Build history of the part. All positions in model axes, mm. A direction names the side the tool comes from. Round coordinates to 2 decimals unless told otherwise and drop trailing zeros. Order: outer loops, then holes, each group sorted by start corner. A loop starts at its lowest first (then second) coordinate and runs counter-clockwise, first axis right, second up. Notation, with made-up numbers: (35, 66) -> (74, 66) arc R18 cw to (74, 78) -> close; hole circle Ø9 at (19.5, 86.25). An arc over 180 degrees is marked (long way). Write item = value, one per line.
from build123d import *

# Parameters (mm, degrees)
SKETCH1_W               = 50
SKETCH1_H               = 18.4
BOSS_EXTRUDE1_DEPTH     = 43
SKETCH2_W               = 7.5
SKETCH2_H               = 5
SKETCH2_W_2             = 30
SKETCH2_H_2             = 1.8
CUT_EXTRUDE1_DEPTH      = 15.6
CUT_EXTRUDE2_START      = -22.5
CUT_EXTRUDE2_DEPTH      = 22.5
CUT_EXTRUDE3_START      = -15
CUT_EXTRUDE3_DEPTH      = 15
BOSS_EXTRUDE3_DEPTH     = 7.5
BOSS_EXTRUDE4_START     = 45
BOSS_EXTRUDE4_DEPTH     = 7.5
BOSS_EXTRUDE7_DEPTH     = 30
MTRL_RMV_DEPTH          = 60.694974663
SKETCH22_W              = 36
SKETCH22_H              = 24.066709319
SKETCH22_W_2            = 3
SKETCH22_H_2            = 2.783290681
BOSS_EXTRUDE8_DEPTH     = 2
BOSS_EXTRUDE9_DEPTH     = 36
SKETCH27_W              = 3
SKETCH27_H              = 21.1
BOSS_EXTRUDE10_DEPTH    = 14.25
SKETCH28_R              = 1.5
CUT_EXTRUDE4_DEPTH      = 53.451549072
SKETCH4_W               = 30
SKETCH4_H               = 11
WIRE_HOLE_DEPTH         = 2.5
SKETCH13_W              = 2
SKETCH13_H              = 2
FRONT_SHIELD_PEGS_DEPTH = 3.175
SKETCH14_W              = 2
SKETCH14_H              = 2
TOP_SHIELD_PEGS_DEPTH   = 3.175
FILLET9_R               = 10
FILLET10_R              = 2
LEGS_START              = 24
LEGS_DEPTH              = 12.7
SKETCH29_W              = 2
SKETCH29_H              = 2
SIDE_SHIELD_PEGS1_DEPTH = 3.175
SIDE_START              = -50
SKETCH29_2_W            = 2
SKETCH29_2_H            = 2
SIDE_SHIELD_PEGS2_DEPTH = 3.175


with BuildPart() as part:
    # Sketch1 → Boss-Extrude1 (new body)
    with BuildSketch(Plane.XY):
        Rectangle(SKETCH1_W, SKETCH1_H)
    extrude(amount=BOSS_EXTRUDE1_DEPTH)

    # Sketch2 → Cut-Extrude1 (cut)
    with BuildSketch(Plane(origin=(0, -9.2, 0), x_dir=(-1, 0, 0), z_dir=(0, -1, 0))):
        with Locations((-18.75, -12)):
            Rectangle(SKETCH2_W, SKETCH2_H)
        with Locations((18.75, -12)):
            Rectangle(SKETCH2_W, SKETCH2_H)
        with Locations((0, -12)):
            Rectangle(SKETCH2_W_2, SKETCH2_H_2)
    extrude(amount=-CUT_EXTRUDE1_DEPTH, mode=Mode.SUBTRACT)

    # Sketch3 → Cut-Extrude2 (cut)
    with BuildSketch(Plane(origin=(0, 0, 0), x_dir=(0, 0, -1), z_dir=(1, 0, 0)).offset(CUT_EXTRUDE2_START)):
        Polygon((-40.5, 6.2), (-40.5, -9.2), (-2.5, -9.2), (-2.5, 6.2), (-11.825335932, -1.144738516), align=None)
    cut_extrude2 = extrude(amount=CUT_EXTRUDE2_DEPTH, mode=Mode.SUBTRACT)

    # Mirror3: Cut-Extrude2 across plane
    add(cut_extrude2.mirror(Plane(origin=(0, 0, 0), x_dir=(0, 0, 1), z_dir=(1, 0, 0))), mode=Mode.SUBTRACT)

    # Sketch3<3> → Cut-Extrude3 (cut)
    with BuildSketch(Plane(origin=(0, 0, 0), x_dir=(0, 0, -1), z_dir=(1, 0, 0)).offset(CUT_EXTRUDE3_START)):
        Polygon((-12, 1.9), (-2.731466864, 9.2), (-40.5, 9.2), (-21.687267414, 4.381300074), (-12, 1.6), align=None)
    cut_extrude3 = extrude(amount=CUT_EXTRUDE3_DEPTH, mode=Mode.SUBTRACT)

    # Mirror4: Cut-Extrude3 across plane
    add(cut_extrude3.mirror(Plane(origin=(0, 0, 0), x_dir=(0, 0, 1), z_dir=(1, 0, 0))), mode=Mode.SUBTRACT)

    # Sketch12 → Boss-Extrude3 (add)
    with BuildSketch(Plane.ZY.offset(-22.5)):
        Polygon((9.5, 6.4), (9.5, 0.686721981), (9.625, 6.4), align=None)
        Polygon((14.5, 6.4), (14.5, 0.686721981), (14.375, 6.4), align=None)
    extrude(amount=BOSS_EXTRUDE3_DEPTH)

    # Sketch12<2> → Boss-Extrude4 (add)
    with BuildSketch(Plane.ZY.offset(-22.5).offset(BOSS_EXTRUDE4_START)):
        Polygon((9.5, 6.4), (9.5, 0.686721981), (9.625, 6.4), align=None)
        Polygon((14.5, 6.4), (14.5, 0.686721981), (14.375, 6.4), align=None)
    extrude(amount=-BOSS_EXTRUDE4_DEPTH)

    # Sketch17 → Boss-Extrude7 (add)
    with BuildSketch(Plane(origin=(-15, 0, 0), x_dir=(0, 0, -1), z_dir=(1, 0, 0))):
        Polygon((-43, 9.2), (-43, 10.7), (-21.687267414, 4.381300074), (-40.5, 9.2), align=None)
    extrude(amount=BOSS_EXTRUDE7_DEPTH)

    # Sketch18 → Mtrl Rmv (cut, through all)
    with BuildSketch(Plane(origin=(15, 0, 0), x_dir=(0, 0, -1), z_dir=(1, 0, 0))):
        Polygon((-43, 10.7), (-43, 9.2), (-37.940557511, 9.2), align=None)
    extrude(amount=-MTRL_RMV_DEPTH, mode=Mode.SUBTRACT)

    # Sketch22 → Boss-Extrude8 (add)
    with BuildSketch(Plane.XY.offset(30.75)):
        with Locations((0, 24.016645341)):
            Rectangle(SKETCH22_W, SKETCH22_H)
        with Locations((16.5, 10.591645341)):
            Rectangle(SKETCH22_W_2, SKETCH22_H_2)
        with Locations((-16.5, 10.591645341)):
            Rectangle(SKETCH22_W_2, SKETCH22_H_2)
    extrude(amount=-BOSS_EXTRUDE8_DEPTH)

    # Sketch25 → Boss-Extrude9 (add)
    with BuildSketch(Plane(origin=(18, 0, 0), x_dir=(0, 0, -1), z_dir=(1, 0, 0))):
        Polygon((-43, 30.3), (-43, 9.2), (-37.940557511, 9.2), (-41.5, 10.25528697), (-41.5, 18.655212051), (-35.764164569, 18.655212051), (-41.5, 23.3), (-41.5, 30.3), align=None)
        Polygon((-30.75, 11.983290681), (-30.75, 18.655212051), (-34.323998772, 11.983290681), align=None)
    extrude(amount=-BOSS_EXTRUDE9_DEPTH)

    # Sketch27 → Boss-Extrude10 (add)
    with BuildSketch(Plane.XY.offset(43)):
        with Locations((-16.5, 19.75)):
            Rectangle(SKETCH27_W, SKETCH27_H)
        with Locations((16.5, 19.75)):
            Rectangle(SKETCH27_W, SKETCH27_H)
    extrude(amount=-BOSS_EXTRUDE10_DEPTH)

    # Sketch28 → Cut-Extrude4 (cut, through all)
    with BuildSketch(Plane(origin=(0, 0, 28.75), x_dir=(-1, 0, 0), z_dir=(0, 0, -1))):
        with Locations((0, 32.8)):
            Circle(SKETCH28_R)
    extrude(amount=-CUT_EXTRUDE4_DEPTH, mode=Mode.SUBTRACT)

    # Sketch4 → Wire Hole (cut)
    with BuildSketch(Plane.XY.offset(43)):
        with Locations((0, -3.7)):
            Rectangle(SKETCH4_W, SKETCH4_H)
    extrude(amount=-WIRE_HOLE_DEPTH, mode=Mode.SUBTRACT)

    # Sketch13 → Front Shield Pegs (add)
    with BuildSketch(Plane(origin=(0, 0, 0), x_dir=(-1, 0, 0), z_dir=(0, 0, -1))):
        with Locations((-14, 0)):
            Rectangle(SKETCH13_W, SKETCH13_H)
        with Locations((14, 0)):
            Rectangle(SKETCH13_W, SKETCH13_H)
    extrude(amount=FRONT_SHIELD_PEGS_DEPTH)

    # Sketch14 → Top Shield Pegs (add)
    with BuildSketch(Plane(origin=(0, 9.2, 0), x_dir=(1, 0, 0), z_dir=(0, 1, 0))):
        with Locations((20, -23)):
            Rectangle(SKETCH14_W, SKETCH14_H)
        with Locations((-20, -23)):
            Rectangle(SKETCH14_W, SKETCH14_H)
    extrude(amount=TOP_SHIELD_PEGS_DEPTH)

    # Fillet9
    # the kernel refuses this fillet: 10 mm, written as the material it takes off along each edge
    with BuildSketch(Plane(origin=(-15, 9.2, 2.731466864), x_dir=(0, 0, -1), z_dir=(1, 0, 0))) as fillet9_piece_1:
        with BuildLine():
            CenterArc((FILLET9_R * 0.346519160452, -FILLET9_R), FILLET9_R, 90, 38.224362431)
            Line((-FILLET9_R * 0.27222332899, -FILLET9_R * 0.214406127977), (0, 0))
            Line((0, 0), (FILLET9_R * 0.346519160452, 0))
        make_face()
    extrude(amount=30, mode=Mode.SUBTRACT)

    # Fillet10
    fillet10_edges = [part.edges().sort_by_distance(p)[0] for p in [
        (0, 2.608850031, 11.1),
    ]]
    fillet(fillet10_edges, radius=FILLET10_R)

    # Sketch19 → Legs (add)
    with BuildSketch(Plane.XY.offset(19).offset(LEGS_START)):
        Polygon((22.5, -9.2), (22.5, -17.915), (29, -17.915), (29, -14.915), (25, -14.915), (25, -9.2), align=None)
        Polygon((-22.5, -9.2), (-22.5, -17.915), (-29, -17.915), (-29, -14.915), (-25, -14.915), (-25, -9.2), align=None)
    extrude(amount=-LEGS_DEPTH)

    # Sketch29 → Side Shield Pegs1 (add)
    with BuildSketch(Plane.ZY.offset(25)):
        with Locations((23, 0)):
            Rectangle(SKETCH29_W, SKETCH29_H)
    extrude(amount=SIDE_SHIELD_PEGS1_DEPTH)

    # Sketch29<2> → Side Shield Pegs2 (add)
    with BuildSketch(Plane.ZY.offset(25).offset(SIDE_START)):
        with Locations((23, 0)):
            Rectangle(SKETCH29_2_W, SKETCH29_2_H)
    extrude(amount=-SIDE_SHIELD_PEGS2_DEPTH)


solid = part.part
Q1. Cut at B-B, the plane x = 0. Give the number of separate pieces and of enclosed holes in the cut face, and give its area (3 significant figures).
Check values:
separate_pieces = 4
enclosed_holes = 0
area = 279 mm²
Q2. Flat gauge pins, fed straight in: pin 1 (2 mm diameter, centred on x = -9.5, y = -7, fed in from -Z); pin 2 (15.5 mm diameter, centred on y = 21, z = 33.5, fed in from -X); pin 3 (4 mm diameter, centred on x = 4.5, z = 9, fed in from +Y). Where does each tip first touch, or does it go through?
Check values:
pin_1 = 0
pin_2 = -18
pin_3 = 5.84
Q3. Cut at C-C, the plane x = 10.5. List the corners of the cut face in (y, z).
Check values:
outline = (-9.2, 0) -> (9.17, 0) arc R10 ccw to (7.06, 5.45) -> (3.21, 10.34) arc R2 ccw to (1.64, 11.1) -> (-0.57, 11.1) -> (6.2, 2.5) -> (-9.2, 2.5) -> close; (-0.87, 12.9) -> (1.86, 12.9) -> (4.38, 21.69) -> (10.26, 41.5) -> (18.66, 41.5) -> (18.66, 35.76) -> (23.3, 41.5) -> (30.3, 41.5) -> (30.3, 43) -> (1.8, 43) -> (1.8, 40.5) -> (6.2, 40.5) -> close; (11.98, 28.75) -> (36.05, 28.75) -> (36.05, 30.75) -> (18.66, 30.75) -> (11.98, 34.32) -> close
Q4. Mould opens along Z. For faces 5 (the face through (-20, 11, 24)), 6 (the face through (-2, -9.2, 2)), 7 (the face through (0.32, 2.86, 6.74)), 8 (the face through (-27, 0, 22)) say: released by +Z, released by -Z, zero draft, split by the parting line, or undercut.
Check values:
face_5 = released by +Z
face_6 = zero draft
face_7 = undercut
face_8 = released by -Z
Q5. Cut at A-A, the plane y = 32.8. List the corners of the cut face in (x, z), and give its area (3 significant figures).
Check values:
outline = (-18, 28.75) -> (-1.5, 28.75) -> (-1.5, 30.75) -> (-18, 30.75) -> close; (1.5, 28.75) -> (18, 28.75) -> (18, 30.75) -> (1.5, 30.75) -> close
area = 66.0 mm²
Q6. Cut at D-D, the plane y = 26. List the corners of the cut face in (x, z).
Check values:
outline = (-18, 28.75) -> (18, 28.75) -> (18, 43) -> (-18, 43) -> close; hole (-15, 30.75) -> (15, 30.75) -> (15, 41.5) -> (-15, 41.5) -> close
Q7. Probe probe 1 along X at (y, z) = (6, 16); probe 2 along Y at (x, z) = (0, 29); probe 3 along Z at (x, y) = (-21.5, -9). List the from-to ranges inside material, lowest first.
Check values:
probe_1 = -25 to -15, 15 to 25
probe_2 = 3.25 to 6.55, 11.98 to 31.3, 34.3 to 36.05
probe_3 = 0 to 2.5, 40.5 to 43
Q8. Which spindle directions (+Z, -Z, +X, -X, +Y, -Y) get a long thin tool onto all of the face, cutting with end or side? Do faces 1 (the face through (0, 18.655, 39)), 2 (the face through (-27, -14.915, 37)), 3 (the face through (0.21, 15.37, 32.51)), 4 (the face through (-15, 2, 10)). Say none if no direction does.
Check values:
face_1 = none
face_2 = +Z, -Z, -X, +Y
face_3 = +Y
face_4 = -Y
